The model under review builds one solid part; all positions refer to its coordinate system, in mm. Face numbers are marked on the shaded views. A direction names the side the tool comes from. Give positions to 0.01 mm unless a question says otherwise; leave off trailing zeros. Order: outer loops, then holes, each group sorted by start corner. A loop starts at its lowest first (then second) coordinate and runs counter-clockwise, first axis right, second up.
```python
from build123d import *

# Parameters (mm, degrees)
F1_DEPTH = 130.175
F2_R     = 23.01875
F3_DEPTH = 25.4


with BuildPart() as f1:
    # F0 (on Front) → F1 (new body)
    with BuildSketch(Plane.XZ):
        Polygon((-38.131632, 38.681432), (-47.656632, 38.681432), (-47.656632, -50.218568), (22.193368, -50.218568), (22.193368, -40.693568), (-38.131632, -40.693568), align=None)
    extrude(amount=F1_DEPTH)

    # F2 (on face) → F3 (cut)
    with BuildSketch(Plane.YZ.offset(-38.131632)):
        Polygon((-130.175, -2.593568), (-92.075, 38.681432), (-130.175, 38.681432), align=None)
        Polygon((-38.1, 38.681432), (0, -2.593568), (0, 0), (0, 38.681432), align=None)
        with Locations((-66.177778, -0.212318)):
            Circle(F2_R)
    extrude(amount=-F3_DEPTH, mode=Mode.SUBTRACT)


solid = f1.part
```
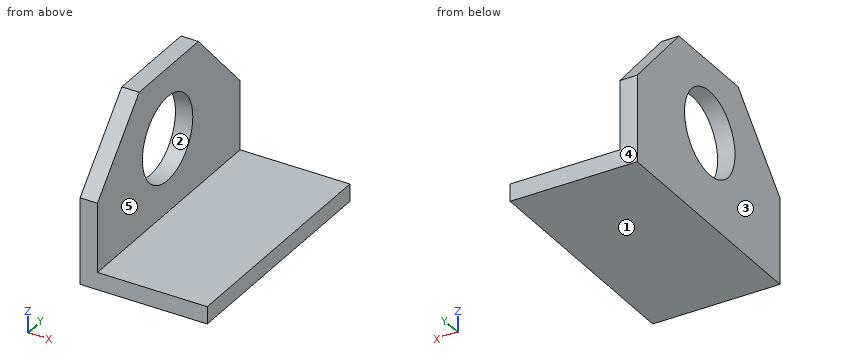
1. For the marked faces 4 and 5, list the 3-axis set-ups (+Z, -Z, +X, -X, +Y, -Y) from which the entire face can be reached by the end or side of a thin tool; tool diameter is ignored.
2. To check wall thickness, follow line 1 (Z direction, x = -31.5, y = -70.5); line 2 (X direction, y = -28.5, z = -36); line 3 (Y direction, x = -39.5, z = -13.5) (1 decimal). State the ranges of each line that lie inside material, in increasing order.
3. Take a section at A-A (z = -15). Write out the cut boundary in (x, y) (3 decimals), and give its area (3 significant figures).
4. Draft analysis for pull direction Z (two halves, no side actions). For the marked faces 1, 2 and 3, state which applies: pulls with the +Z half, pulls with the -Z half, needs draft (parallel to the pull), parting line crosses it, or undercut.
5. Take a section at B-B (x = -41). Write out the cut boundary in (y, z) (1 decimal), and give its area (3 significant figures).
6. Take a section at C-C (y = -46.5). Write out the cut boundary in (x, z), and give its area (3 significant figures).
7. Take a section at D-D (x = 8). Write out the cut boundary in (y, z) (3 decimals), and give its area (3 significant figures).
8. Insertion check: pin 1 (2 mm diameter, centred on y = -85, z = 7.5, fed in from +X); pin 2 (6 mm diameter, centred on x = -37.5, z = -3.5, fed in from +Y); pin 3 (2 mm diameter, centred on y = -104.5, z = 9, fed in from +X); pin 4 (2 mm diameter, centred on x = 8.5, y = -30.5, fed in from +Z). Each pin has a flat end and moves straight along its axis. Give the tip position at first contact, or say it passes through.
Answer:
1. face 4: +Z, -Z, +X, -X, +Y
1. face 5: +Z, +X, +Y, -Y
2. line 1: z = -50.22 to -40.69
2. line 2: x = -47.66 to -38.13
2. line 3: y = -130.2 to -85, -47.4 to 0
3. outline: (-47.657, -130.175) - (-38.132, -130.175) - (-38.132, -83.818) - (-47.657, -83.818) - close; (-47.657, -48.537) - (-38.132, -48.537) - (-38.132, 0) - (-47.657, 0) - close
3. area: 904 mm2
4. face 1: pulls with the -Z half
4. face 2: undercut
4. face 3: needs draft
5. outline: (-130.2, -50.2) - (0, -50.2) - (0, -2.6) - (-38.1, 38.7) - (-92.1, 38.7) - (-130.2, -2.6) - close; hole circle Ø46 at (-66.2, -0.2)
5. area: 8,340 mm2
6. outline: (-47.66, -50.22) - (22.19, -50.22) - (22.19, -40.69) - (-38.13, -40.69) - (-38.13, -12.16) - (-47.66, -12.16) - close; (-47.66, 11.73) - (-38.13, 11.73) - (-38.13, 38.68) - (-47.66, 38.68) - close
6. area: 1,190 mm2
7. outline: (-130.175, -50.219) - (0, -50.219) - (0, -40.694) - (-130.175, -40.694) - close
7. area: 1,240 mm2
8. pin 1: passes through
8. pin 2: stops at y = 0
8. pin 3: stops at x = -38.13
8. pin 4: stops at z = -40.69
